```python
from build123d import *

# Parameters (mm, degrees)
F0_W     = 144
F0_H     = 154
F1_DEPTH = 44
F2_W     = 15
F2_H     = 9
F2_W_2   = 13
F2_W_3   = 4
F2_H_2   = 13
F3_DEPTH = 2
F4_R     = 1.5


with BuildPart() as f1:
    # F0 (on Top) → F1 (new body)
    with BuildSketch(Plane.XY):
        Rectangle(F0_W, F0_H)
    extrude(amount=F1_DEPTH)

    # F2 (on face) → F3 (cut)
    with BuildSketch(Plane.YZ.offset(72)):
        with Locations((-55.5, 10)):
            Rectangle(F2_W, F2_H)
        with Locations((-39, 10)):
            Rectangle(F2_W, F2_H)
        with Locations((-13, 10)):
            Rectangle(F2_W_2, F2_H)
        with Locations((1.5, 10)):
            Rectangle(F2_W_2, F2_H)
        with Locations((26.5, 10)):
            Rectangle(F2_W_2, F2_H)
        with Locations((41, 10)):
            Rectangle(F2_W_2, F2_H)
        with Locations((59.5, 12.5)):
            Rectangle(F2_W_3, F2_H_2)
    extrude(amount=-F3_DEPTH, mode=Mode.SUBTRACT)

    # F4
    f4_edges = [f1.edges().sort_by_distance(p)[0] for p in [
        (0, -77, 44),
        (0, 77, 44),
        (0, -77, 0),
        (0, 77, 0),
    ]]
    fillet(f4_edges, radius=F4_R)


solid = f1.part
```
Design review of the part built by this model. Coordinates are the model's own, in mm. A direction names the side the tool comes from. Round coordinates to 2 decimals unless told otherwise and drop trailing zeros. Answer in a Markdown table with one row per item.
Q1. To check wall thickness, follow L1, parallel to X at y = -44.5, z = 12. State the ranges of the line that lie inside material, in increasing order. Write a range as [from, to].
The answers:
| item | result |
|---|---|
| L1 | [-72, 70] |
Q2. Draft analysis for pull direction Z (two halves, no side actions). For faces 3 (the face through (70, -39, 10)), 4 (the face through (72, -1, 22)), 5 (the face through (-1, 1, 0)), state which applies: +Z half, -Z half, draft (parallel to the pull), parting line (faces both ways), or undercut.
The answers:
| item | result |
|---|---|
| face 3 | undercut |
| face 4 | draft |
| face 5 | -Z half |
Q3. For faces 1 (the face through (-1, 77, 22)), 2 (the face through (70, 41, 10)), list the 3-axis set-ups (+Z, -Z, +X, -X, +Y, -Y) from which the entire face can be reached by the end or side of a thin tool; tool diameter is ignored.
The answers:
| item | result |
|---|---|
| face 1 | +Z, -Z, +X, -X, +Y |
| face 2 | +X |
Q4. Clearance check with a flat-ended pin moving along its axis: pin 1 Ø4.5 at (y, z) = (4, 8) entering from +X. State where the tip first meets the part, or that it passes through.
The answers:
| item | result |
|---|---|
| pin 1 | x = 70 |
